from build123d import *

# Parameters (mm, degrees)
EXTRUDE_1_DEPTH = 23
SKETCH_2_R      = 3.9
EXTRUDE_2_DEPTH = 20


with BuildPart() as part:
    # 草图1 → 凸台-拉伸1 (new body)
    with BuildSketch(Plane.XY):
        with BuildLine():
            Line((-1.4, 3.640054945), (-1.4, 4.4))
            Line((-1.4, 4.4), (1.3, 4.4))
            Line((1.3, 4.4), (1.3, 3.676955262))
            ThreePointArc((1.3, 3.676955262), (0.053295482, -3.899635828), (-1.4, 3.640054945))
        make_face()
    extrude(amount=EXTRUDE_1_DEPTH)

    # 草图2 → 凸台-拉伸2 (add)
    with BuildSketch(Plane.XY.offset(23)):
        with Locations(Location((0, 0, 0), (0, 0, 111.037221256))):
            Circle(SKETCH_2_R)
    extrude(amount=EXTRUDE_2_DEPTH)


solid = part.part
The listing builds one solid part. Answer for the finished solid, in the listing's coordinates (mm). Round coordinates to 2 decimals unless told otherwise and drop trailing zeros. Write each loop counter-clockwise with the first axis right and the second up, starting at its lowest first coordinate (ties: lowest second). Pieces come first, ordered by that corner, then holes. Notation, with made-up numbers: (-25.75, -12) - (-15.75, -12) arc R23 cw to (-15.75, 4) - close; hole circle Ø6 at (16.25, 1). An arc over 180 degrees is marked (long way). Use a Markdown table: item, result. Add a question column.
1. The part is cut by section C-C (z = 40). Write down the section's boundary in (x, y).
2. The part is cut by section A-A (x = 0). Write down the section's boundary in (y, z).
3. The part is cut by section D-D (x = 2). Write down the section's boundary in (y, z).
4. Flat-ended cylindrical pins translate along their axes: P1, Ø1, axis at y = -1.5, z = 33.5, coming from the +X side; P2, Ø1, axis at y = -1, z = 32.5, coming from the -X side. Find the tip coordinate at first contact, or state that the pin passes through.
5. The part is cut by section B-B (y = -1). Write down the section's boundary in (x, z), and give its area (3 significant figures).
6. Consider line 1 (X direction, y = 3.75, z = 12.5); line 2 (X direction, y = 0.25, z = 32.5); line 3 (Y direction, x = 0, z = 33). Determine where each line is inside the solid, lowest interval first.
Reported:
| question | item | result |
|---|---|---|
| 1 | outline | circle Ø7.8 at (0, 0) |
| 2 | outline | (-3.9, 0) - (4.4, 0) - (4.4, 23) - (3.9, 23) - (3.9, 43) - (-3.9, 43) - close |
| 3 | outline | (-3.35, 0) - (3.35, 0) - (3.35, 43) - (-3.35, 43) - close |
| 4 | P1 | x = 3.77 |
| 4 | P2 | x = -3.87 |
| 5 | outline | (-3.77, 0) - (3.77, 0) - (3.77, 43) - (-3.77, 43) - close |
| 5 | area | 324 mm^2 |
| 6 | line 1 | -1.4 to 1.3 |
| 6 | line 2 | -3.89 to 3.89 |
| 6 | line 3 | -3.9 to 3.9 |
